Check sheet for the modelled part. Datum: model origin and axes. Units: mm. Face numbers are marked on the shaded views. A direction names the side the tool comes from. Coordinates: 2 decimals unless noted, no trailing zeros. Write each loop counter-clockwise with the first axis right and the second up, starting at its lowest first coordinate (ties: lowest second). Pieces come first, ordered by that corner, then holes. Notation, with made-up numbers: (-20, 22.25) - (23, 22.25) arc R12 ccw to (23, 32.25) - close; hole circle Ø2 at (9.5, 14.5). An arc over 180 degrees is marked (long way). Answer as CSV lines item,"result". Start each with the question number.
from build123d import *

# Parameters (mm, degrees)
PAD_DEPTH       = 3
SKETCH001_R     = 11
PAD001_DEPTH    = 3
SKETCH002_R     = 10.1
POCKET_DEPTH    = 5.1
SKETCH003_R     = 1.7
POCKET001_DEPTH = 5


with BuildPart() as part:
    # Sketch → Pad (new body)
    with BuildSketch(Plane.XY):
        Polygon((-12.5, -5), (-22.5, -5), (-22.5, 5), (-12.5, 5), (-12.5, 12), (12.5, 12), (12.5, 5), (22.5, 5), (22.5, -5), (12.5, -5), (12.5, -12), (-12.5, -12), align=None)
    extrude(amount=PAD_DEPTH)

    # Sketch001 (on Face13 of Pad) → Pad001 (join)
    with BuildSketch(Plane(origin=(0, 0, 0), x_dir=(1, 0, 0), z_dir=(0, 0, -1))):
        Circle(SKETCH001_R)
    extrude(amount=PAD001_DEPTH)

    # Sketch002 (on Face5 of Pad001) → Pocket (cut)
    with BuildSketch(Plane.XY.offset(3)):
        Circle(SKETCH002_R)
    extrude(amount=-POCKET_DEPTH, mode=Mode.SUBTRACT)

    # Sketch003 (on Face5 of Pocket) → Pocket001 (cut)
    with BuildSketch(Plane.XY.offset(3)):
        with Locations((-17.5, 0)):
            Circle(SKETCH003_R)
        with Locations((17.5, 0)):
            Circle(SKETCH003_R)
    extrude(amount=-POCKET001_DEPTH, mode=Mode.SUBTRACT)


solid = part.part
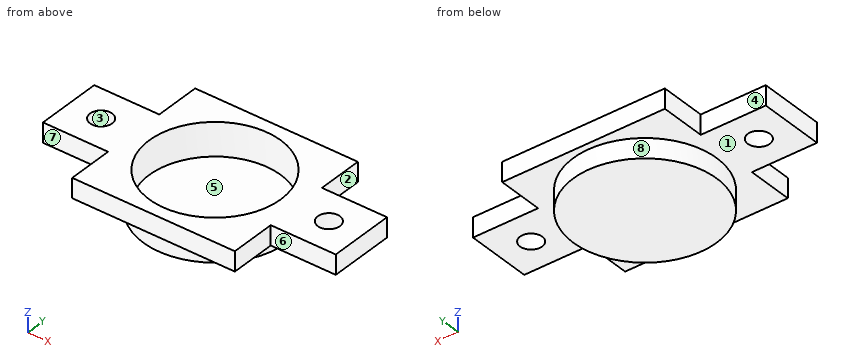
(1) Cross-section at B-B on y = 0. Record the boundary of the cut face in (x, z).
(2) Cross-section at D-D on y = 4.5. Record the boundary of the cut face in (x, z).
(3) Cross-section at C-C on x = 0. Record the boundary of the cut face in (y, z), plus the area to 3 significant figures.
(4) Cross-section at A-A on x = 17.5. Record the boundary of the cut face in (y, z), plus the area to 3 significant figures.
(5) Go/stop test with flat-tipped pins: P1, Ø2.5, axis at x = -19.5, z = 1, coming from the -Y side; P2, Ø6, axis at x = 3.5, y = 8.5, coming from the +Z side; P3, Ø6, axis at x = -12.5, y = -7, coming from the -Z side; P4, Ø1.5, axis at y = 7, z = 2, coming from the +X side. Record where each tip stops, or that it passes through.
(6) Release check for a two-part mould opening along X. For the marked faces 1, 2 and 3 record: pulls with the +X half, pulls with the -X half, needs draft (parallel to the pull), parting line crosses it, or undercut.
(7) Material ranges on probe 1 along Y at (x, z) = (0, -1.6); probe 2 along Y at (x, z) = (17.5, 2.45); probe 3 along Z at (x, y) = (-13, -1.5), recorded low to high. Write a range as from..to.
(8) Tool access check on the marked faces 4, 5, 6, 7 and 8. Record the directions out of +Z, -Z, +X, -X, +Y, -Y that give a thin tool (end or side, any length) a straight path to the whole face; none if there is none.
Checked values:
1,outline,"(-22.5, 0) - (-19.2, 0) - (-19.2, 3) - (-22.5, 3) - close; (-15.8, 0) - (-11, 0) - (-11, -3) - (11, -3) - (11, 0) - (15.8, 0) - (15.8, 3) - (10.1, 3) - (10.1, -2.1) - (-10.1, -2.1) - (-10.1, 3) - (-15.8, 3) - close; (19.2, 0) - (22.5, 0) - (22.5, 3) - (19.2, 3) - close"
2,outline,"(-22.5, 0) - (-10.04, 0) - (-10.04, -3) - (10.04, -3) - (10.04, 0) - (22.5, 0) - (22.5, 3) - (9.04, 3) - (9.04, -2.1) - (-9.04, -2.1) - (-9.04, 3) - (-22.5, 3) - close"
3,outline,"(-12, 0) - (-11, 0) - (-11, -3) - (11, -3) - (11, 0) - (12, 0) - (12, 3) - (10.1, 3) - (10.1, -2.1) - (-10.1, -2.1) - (-10.1, 3) - (-12, 3) - close"
3,area,"35.0 mm^2"
4,outline,"(-5, 0) - (-1.7, 0) - (-1.7, 3) - (-5, 3) - close; (1.7, 0) - (5, 0) - (5, 3) - (1.7, 3) - close"
4,area,"19.8 mm^2"
5,P1,"y = -5"
5,P2,"z = 3"
5,P3,"z = 0"
5,P4,"x = 12.5"
6,face 1,"needs draft"
6,face 2,"pulls with the +X half"
6,face 3,"undercut"
7,probe 1,"-11..-10.1, 10.1..11"
7,probe 2,"-5..-1.7, 1.7..5"
7,probe 3,"0..3"
8,face 4,"+Z, -Z, -X, +Y"
8,face 5,"+Z"
8,face 6,"+Z, -Z, +X, -Y"
8,face 7,"+Z, -Z, -X, -Y"
8,face 8,"-Z"
